```python
from build123d import *

# Parameters (mm, degrees)
SKETCH2_R           = 3
SKETCH2_R_2         = 5
BOSS_EXTRUDE1_DEPTH = 6
SKETCH4_R           = 6.5
CUT_EXTRUDE1_DEPTH  = 4


with BuildPart() as part:
    # Sketch2 → Boss-Extrude1 (new body)
    with BuildSketch(Plane(origin=(0, 0, 0), x_dir=(1, 0, 0), z_dir=(0, 1, 0))):
        with BuildLine():
            Line((-6.5, 28.5), (123.5, 28.5))
            ThreePointArc((123.5, 28.5), (138.5, 13.5), (123.5, -1.5))
            Line((123.5, -1.5), (-6.5, -1.5))
            ThreePointArc((-6.5, -1.5), (-21.5, 13.5), (-6.5, 28.5))
        make_face()
        with Locations(Location((-6.5, 13.5, 0), (0, 0, 270))):
            Circle(SKETCH2_R, mode=Mode.SUBTRACT)
        with Locations(Location((123.5, 13.5, 0), (0, 0, 270))):
            Circle(SKETCH2_R_2, mode=Mode.SUBTRACT)
    extrude(amount=BOSS_EXTRUDE1_DEPTH)

    # Sketch4 → Cut-Extrude1 (cut)
    with BuildSketch(Plane.XZ):
        with Locations(Location((123.5, -13.5, 0), (0, 0, 270))):
            Circle(SKETCH4_R)
    extrude(amount=-CUT_EXTRUDE1_DEPTH, mode=Mode.SUBTRACT)


solid = part.part
```
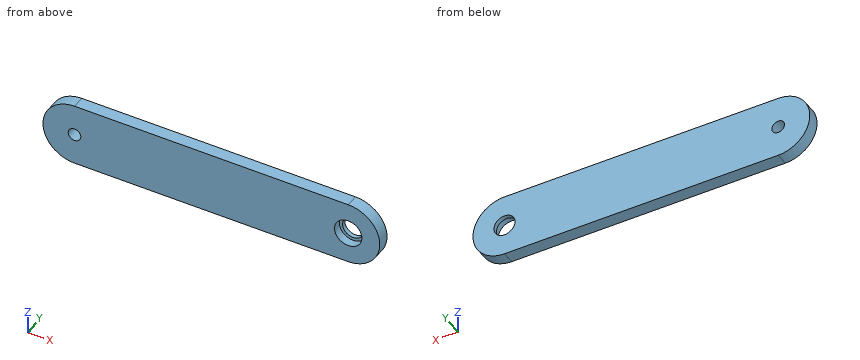
Input: part model. Units: mm. Frame: model coordinates. Coordinates: 2 decimals unless noted, no trailing zeros. Loops run counter-clockwise (first coordinate to the right, second up) from the corner with the lowest first, then second, coordinate; pieces in that order, holes last. Notation, with made-up numbers: M -13.75,52.25 L 11.25,52.25 A18 cw 11.25,60.25 Z; hole C -25.5,83 d1. An arc over 180 degrees is marked long. Use a Markdown table: item, result. Add a question column.
1) Line query: L1, parallel to X at y = 1.3, z = -13.5; L2, parallel to X at y = 4.65, z = -13.5; L3, parallel to Z at x = 120.5, y = 5.1. Output: solid intervals per line, ascending. Write a range as from..to.
2) Section C-C, the plane z = -24. Return the cut outline in (x, y).
3) Section B-B, the plane y = 3.1. Return the cut outline in (x, z), plus the area to 3 significant figures.
4) Section A-A, the plane z = -13.5. Return the cut outline in (x, y).
5) Section D-D, the plane z = -4. Return the cut outline in (x, y), plus the area to 3 significant figures.
6) Pin query (flat end, axial travel): P1, Ø5.5, axis at x = -6.5, z = -13.5, coming from the -Y side; P2, Ø6.5, axis at x = 125, z = -15, coming from the -Y side. Return the tip coordinate at first contact, or that it passes through.
Answer below:
| question | item | result |
|---|---|---|
| 1 | L1 | -21.5..-9.5, -3.5..117, 130..138.5 |
| 1 | L2 | -21.5..-9.5, -3.5..118.5, 128.5..138.5 |
| 1 | L3 | -28.5..-17.5, -9.5..1.5 |
| 2 | outline | M -17.21,0 L 134.21,0 L 134.21,6 L -17.21,6 Z |
| 3 | outline | M -6.5,-28.5 L 123.5,-28.5 A15 ccw 123.5,1.5 L -6.5,1.5 A15 ccw Z; hole C -6.5,-13.5 d6; hole C 123.5,-13.5 d13 |
| 3 | area | 4,450 mm2 |
| 4 | outline | M -21.5,0 L -9.5,0 L -9.5,6 L -21.5,6 Z; M -3.5,0 L 117,0 L 117,4 L 118.5,4 L 118.5,6 L -3.5,6 Z; M 128.5,4 L 130,4 L 130,0 L 138.5,0 L 138.5,6 L 128.5,6 Z |
| 5 | outline | M -18.11,0 L 135.11,0 L 135.11,6 L -18.11,6 Z |
| 5 | area | 919 mm2 |
| 6 | P1 | through |
| 6 | P2 | y = 4 |
